Check sheet for the modelled part. Datum: model origin and axes. Units: mm. Face numbers are marked on the shaded views. A direction names the side the tool comes from. Give positions to 0.01 mm unless a question says otherwise; leave off trailing zeros. Order: outer loops, then holes, each group sorted by start corner. A loop starts at its lowest first (then second) coordinate and runs counter-clockwise, first axis right, second up. Notation, with made-up numbers: (-9.75, 31) -> (15.25, 31) arc R5 ccw to (15.25, 36) -> close; hole circle Ø5 at (39.5, -33). An arc over 180 degrees is marked (long way). Answer in a Markdown table with one row per item. Add a question column.
(1) Cross-section at B-B (x = -42). Record the cut outline in (y, z), then the cut area to 3 significant figures.
(2) Cross-section at C-C (y = 6). Record the cut outline in (x, z).
(3) Cross-section at A-A (y = 38). Record the cut outline in (x, z).
(4) Cross-section at D-D (z = -35). Record the cut outline in (x, y).
(5) Go/stop test with flat-tipped pins: pin 1 (8 mm diameter, centred on y = 16.5, z = -23, fed in from +X); pin 2 (1.5 mm diameter, centred on x = 34, z = -13.5, fed in from +Y); pin 3 (11.5 mm diameter, centred on y = 30.5, z = -29.5, fed in from -X); pin 4 (11 mm diameter, centred on x = -38, z = -31, fed in from +Y). Record where each tip stops, or that it passes through.
(6) Release check for a two-part mould opening along Y. For the marked faces 1, 2 and 3 record: released by +Y, released by -Y, zero draft, split by the parting line, or undercut.
(7) Thickness scan on L1, parallel to X at y = 6, z = -31; L2, parallel to X at y = 25.5, z = -9; L3, parallel to Z at x = -38, y = 5.25. Record the ranges inside material, lowest first. Write a range as [from, to].
(8) Set-up check for the marked faces 4, 5, 6 and 7: record each of +Z, -Z, +X, -X, +Y, -Y from which the full face is reachable in a straight line by a thin tool's end or side.
```python
from build123d import *

# Parameters (mm, degrees)
SKETCH_2_W          = 114
SKETCH_2_H          = 50
EXTRUDE_1_DEPTH     = 11
FILLET_1_R          = 19
SKETCH_3_W          = 114
SKETCH_3_H          = 11
EXTRUDE_2_DEPTH     = 65
FILLET_2_R          = 19
SKETCH_4_R          = 6
CUT_EXTRUDE_1_DEPTH = 66
CUT_EXTRUDE_3_DEPTH = 65
EXTRUDE_3_DEPTH     = 3


with BuildPart() as part:
    # 스케치2 → 보스-돌출1 (new body)
    with BuildSketch(Plane(origin=(0, 0, 0), x_dir=(1, 0, 0), z_dir=(0, 1, 0))):
        with Locations((0, 25)):
            Rectangle(SKETCH_2_W, SKETCH_2_H)
    extrude(amount=EXTRUDE_1_DEPTH)

    # 필렛1
    fillet_1_edges = [part.edges().sort_by_distance(p)[0] for p in [
        (-57, 5.5, -50),
        (57, 5.5, -50),
    ]]
    fillet(fillet_1_edges, radius=FILLET_1_R)

    # 스케치3 → 보스-돌출2 (add)
    with BuildSketch(Plane(origin=(0, 0, 0), x_dir=(1, 0, 0), z_dir=(0, 1, 0))):
        with Locations((0, 5.5)):
            Rectangle(SKETCH_3_W, SKETCH_3_H)
    extrude(amount=EXTRUDE_2_DEPTH)

    # 필렛2
    fillet_2_edges = [part.edges().sort_by_distance(p)[0] for p in [
        (57, 65, -5.5),
        (-57, 65, -5.5),
    ]]
    fillet(fillet_2_edges, radius=FILLET_2_R)

    # 스케치4 → 컷-돌출1 (cut, through all)
    with BuildSketch(Plane(origin=(0, 0, 0), x_dir=(1, 0, 0), z_dir=(0, 1, 0))):
        with Locations((-38, 31)):
            Circle(SKETCH_4_R)
        with Locations((38, 31)):
            Circle(SKETCH_4_R)
    extrude(amount=CUT_EXTRUDE_1_DEPTH, mode=Mode.SUBTRACT)

    # 스케치5 → 컷-돌출3 (cut)
    with BuildSketch(Plane.XY):
        with BuildLine():
            Line((-44, 46), (-44, 27))
            ThreePointArc((-44, 27), (-38, 21), (-32, 27))
            Line((-32, 27), (-32, 46))
            ThreePointArc((-32, 46), (-38, 52), (-44, 46))
        make_face()
        with BuildLine():
            Line((32, 46), (32, 27))
            ThreePointArc((32, 27), (38, 21), (44, 27))
            Line((44, 27), (44, 46))
            ThreePointArc((44, 46), (38, 52), (32, 46))
        make_face()
    extrude(amount=-CUT_EXTRUDE_3_DEPTH, mode=Mode.SUBTRACT)

    # 스케치9 → 보스-돌출3 (add, symmetric)
    with BuildSketch(Plane(origin=(0, 0, 0), x_dir=(0, 0, -1), z_dir=(1, 0, 0))):
        Polygon((0, 65), (11, 65), (50, 11), (50, 0), (0, 0), align=None)
    extrude(amount=EXTRUDE_3_DEPTH, both=True)


solid = part.part
```
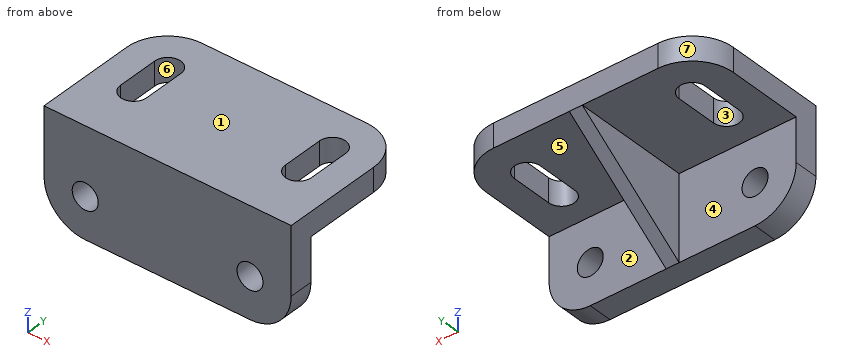
Answer below:
| question | item | result |
|---|---|---|
| 1 | outline | (0, -49.57) -> (11, -49.57) -> (11, -35.47) -> (0, -35.47) -> close; (0, -26.53) -> (11, -26.53) -> (11, -11) -> (22.53, -11) -> (22.53, 0) -> (0, 0) -> close; (50.47, -11) -> (64.57, -11) -> (64.57, 0) -> (50.47, 0) -> close |
| 1 | area | 729 mm² |
| 2 | outline | (-57, -31) arc R19 ccw to (-38, -50) -> (38, -50) arc R19 ccw to (57, -31) -> (57, 0) -> (-57, 0) -> close; hole circle Ø12 at (-38, -31); hole circle Ø12 at (38, -31) |
| 3 | outline | (-57, -11) -> (-44, -11) -> (-44, 0) -> (-57, 0) -> close; (-32, -11) -> (-3, -11) -> (-3, -30.5) -> (3, -30.5) -> (3, -11) -> (32, -11) -> (32, 0) -> (-32, 0) -> close; (44, -11) -> (57, -11) -> (57, 0) -> (44, 0) -> close |
| 4 | outline | (-56.57, 0) -> (-42.47, 0) -> (-42.47, 11) -> (-56.57, 11) -> close; (-33.53, 0) -> (33.53, 0) -> (33.53, 11) -> (3, 11) -> (3, 31.77) -> (-3, 31.77) -> (-3, 11) -> (-33.53, 11) -> close; (42.47, 0) -> (56.57, 0) -> (56.57, 11) -> (42.47, 11) -> close |
| 5 | pin 1 | stops at x = 3 |
| 5 | pin 2 | stops at y = 11 |
| 5 | pin 3 | stops at x = -3 |
| 5 | pin 4 | passes through |
| 6 | face 1 | zero draft |
| 6 | face 2 | released by +Y |
| 6 | face 3 | undercut |
| 7 | L1 | x = [-57, -44], [-32, 32], [44, 57] |
| 7 | L2 | x = [-57, -43.81], [-32.19, 32.19], [43.81, 57] |
| 7 | L3 | z = [-50, -37], [-25, 0] |
| 8 | face 4 | -Z, -X, +Y |
| 8 | face 5 | -Z, +X, +Y |
| 8 | face 6 | +Z, -Z |
| 8 | face 7 | +Z, -Z, -X, +Y |
